from build123d import *

# Parameters (mm, degrees)
SKETCH1_R           = 25
BOSS_EXTRUDE1_DEPTH = 8
BOSS_EXTRUDE2_DEPTH = 20.6


with BuildPart() as part:
    # Sketch1 → Boss-Extrude1 (new body)
    with BuildSketch(Plane(origin=(0, 0, 0), x_dir=(0, 1, 0), z_dir=(0, 0, 1))):
        with Locations(Location((0, 0, 0), (0, 0, 270))):
            Circle(SKETCH1_R)
    extrude(amount=BOSS_EXTRUDE1_DEPTH)

    # Sketch2 → Boss-Extrude2 (add)
    with BuildSketch(Plane.XY.offset(8)):
        with BuildLine():
            Line((-1.715143801, 4.696624505), (-1.715143801, 5.696624505))
            Line((-1.715143801, 5.696624505), (1.715143801, 5.696624505))
            Line((1.715143801, 5.696624505), (1.715143801, 4.696624505))
            ThreePointArc((1.715143801, 4.696624505), (5, 0), (1.715143801, -4.696624505))
            Line((1.715143801, -4.696624505), (1.715143801, -5.696624505))
            Line((1.715143801, -5.696624505), (-1.715143801, -5.696624505))
            Line((-1.715143801, -5.696624505), (-1.715143801, -4.696624505))
            ThreePointArc((-1.715143801, -4.696624505), (-5, 0), (-1.715143801, 4.696624505))
        make_face()
    extrude(amount=BOSS_EXTRUDE2_DEPTH)


solid = part.part
Check sheet for the modelled part. Datum: model origin and axes. Units: mm. A direction names the side the tool comes from. Round coordinates to 2 decimals unless told otherwise and drop trailing zeros. Loops run counter-clockwise (first coordinate to the right, second up) from the corner with the lowest first, then second, coordinate; pieces in that order, holes last. Notation, with made-up numbers: M 69.5,74 L 84.5,74 A19 cw 84.5,100 Z; hole C 18.5,-1.75 d5. An arc over 180 degrees is marked long. One line per question, with ' | ' between items. Start each with the question number.
Item 1: Gauge pin test, flat ends, axial feed: pin 1 Ø1.1 at (y, z) = (5, 19) entering from -X; pin 2 Ø6 at (x, z) = (-7.5, 21.5) entering from +Y; pin 3 Ø6 at (y, z) = (-2.5, 19.5) entering from +X. Record the tip position at first contact, or that the pin passes through.
Item 2: Section check C-C (y = -7). Record the boundary of the cut face in (x, z), and give its area (3 significant figures).
Item 3: Section check D-D (z = 3). Record the boundary of the cut face in (x, y).
Item 4: Section check B-B (z = 15). Record the boundary of the cut face in (x, y).
Item 5: Set-up check for faces 1 (the face through (0, 5.697, 18)), 2 (the face through (-5, 0, 18)), 3 (the face through (0, -5.697, 18)): record each of +Z, -Z, +X, -X, +Y, -Y from which the full face is reachable in a straight line by a thin tool's end or side.
Item 6: Scan lines: probe 1 along Z at (x, y) = (1, 6.5); probe 2 along Y at (x, z) = (0.5, 3) (3 decimals); probe 3 along Y at (x, z) = (-21, 7). Record each from-to range of solid material in increasing order.
Item 7: Section check A-A (y = 0). Record the boundary of the cut face in (x, z).
Worked out:
1) pin 1: x = -2.28 | pin 2: y = 2.18 | pin 3: x = 5
2) outline: M -24,0 L 24,0 L 24,8 L -24,8 Z | area: 384 mm^2
3) outline: C 0,0 d50
4) outline: M -1.72,-5.7 L 1.72,-5.7 L 1.72,-4.7 A5 ccw 1.72,4.7 L 1.72,5.7 L -1.72,5.7 L -1.72,4.7 A5 ccw -1.72,-4.7 Z
5) face 1: +Z, +X, -X, +Y | face 2: +Z, -X | face 3: +Z, +X, -X, -Y
6) probe 1: 0 to 8 | probe 2: -24.995 to 24.995 | probe 3: -13.56 to 13.56
7) outline: M -25,0 L 25,0 L 25,8 L 5,8 L 5,28.6 L -5,28.6 L -5,8 L -25,8 Z
